Can you work these out from the drawing? Everything is in mm from the part's minimum corner. A direction names the side the tool comes from. Give positions to 0.01 mm unless a question says otherwise; leave off trailing zeros. Write each loop counter-clockwise with the first axis right and the second up, starting at its lowest first coordinate (ties: lowest second). Pieces come first, ordered by that corner, then holes. Notation, with made-up numbers: (-30.75, 9.5) - (-0.75, 9.5) arc R21 cw to (-0.75, 24.5) - close; hole circle Ø7 at (81, 30.5). An arc over 180 degrees is marked (long way). Use a Markdown table: item, result.
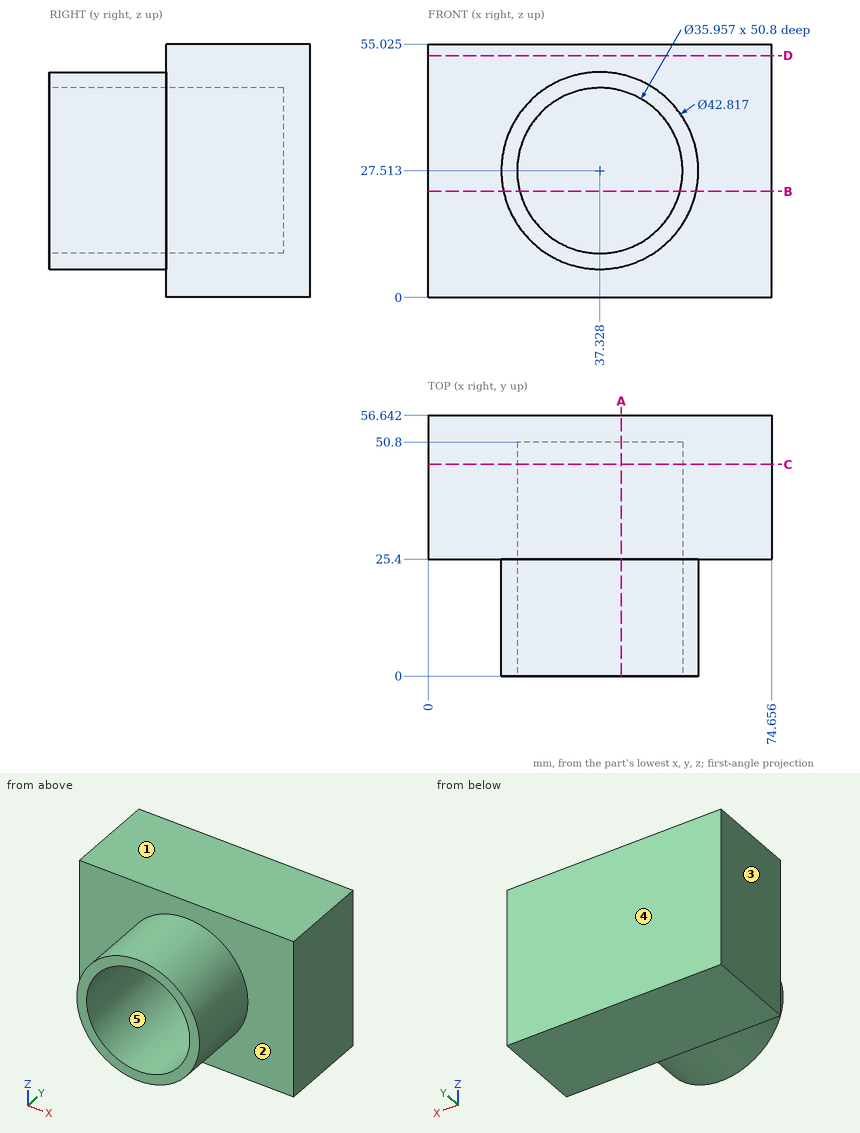
Item 1: Will this pin go through, and if not, where does the flat tip stop? pin 1 Ø10 at (x, y) = (30.5, 11) entering from +Z.
Values:
| item | result |
|---|---|
| pin 1 | stops at z = 48.84 |
Item 2: If we section it at A-A, the plane x = 42: Write out the boundary of the cut face in (y, z) (1 decimal), plus the area to 3 significant figures.
Values:
| item | result |
|---|---|
| outline | (0, 6.6) - (25.4, 6.6) - (25.4, 0) - (56.6, 0) - (56.6, 55) - (25.4, 55) - (25.4, 48.4) - (0, 48.4) - (0, 44.9) - (50.8, 44.9) - (50.8, 10.2) - (0, 10.2) - close |
| area | 1,020 mm2 |
Item 3: I need wall thicknesses on line 1 along Z through (x, y) = (39, 49.5) (1 decimal); line 2 along X through (y, z) = (29, 20) (1 decimal); line 3 along Y through (x, z) = (36, 37). Which ranges of each line are inside material? Lowest first, please. Write a range as [from, to].
Values:
| item | result |
|---|---|
| line 1 | z = [0, 9.6], [45.4, 55] |
| line 2 | x = [0, 21], [53.7, 74.7] |
| line 3 | y = [50.8, 56.64] |
Item 4: If we section it at C-C, the plane y = 46: Write out the boundary of the cut face in (x, z) (1 decimal), plus the area to 3 significant figures.
Values:
| item | result |
|---|---|
| outline | (0, 0) - (74.7, 0) - (74.7, 55) - (0, 55) - close; hole circle Ø36 at (37.3, 27.5) |
| area | 3,090 mm2 |
Item 5: For the marked faces 1 and 2, which set-ups out of +Z, -Z, +X, -X, +Y, -Y let a thin tool reach every point of the face, with its end or its side?
Values:
| item | result |
|---|---|
| face 1 | +Z, +X, -X, +Y, -Y |
| face 2 | -Y |
Item 6: Thinking about a two-plate mould opening in X: for the marked faces 3, 4 and 5, which applies, +X half, -X half, draft (parallel to the pull), parting line (faces both ways), or undercut?
Values:
| item | result |
|---|---|
| face 3 | -X half |
| face 4 | draft |
| face 5 | undercut |
Item 7: If we section it at D-D, the plane z = 52.5: Write out the boundary of the cut face in (x, y).
Values:
| item | result |
|---|---|
| outline | (0, 25.4) - (74.66, 25.4) - (74.66, 56.64) - (0, 56.64) - close |
Item 8: If we section it at B-B, the plane z = 23: Write out the boundary of the cut face in (x, y) (1 decimal).
Values:
| item | result |
|---|---|
| outline | (0, 25.4) - (16.4, 25.4) - (16.4, 0) - (19.9, 0) - (19.9, 50.8) - (54.7, 50.8) - (54.7, 0) - (58.3, 0) - (58.3, 25.4) - (74.7, 25.4) - (74.7, 56.6) - (0, 56.6) - close |
